Geometry check sheet. Reference: the model listing, model coordinates, mm. Face numbers are marked on the shaded views. Give positions to 0.01 mm unless a question says otherwise; leave off trailing zeros. Loops run counter-clockwise (first coordinate to the right, second up) from the corner with the lowest first, then second, coordinate; pieces in that order, holes last. Notation, with made-up numbers: (25, 20) -> (37, 20) arc R24 cw to (37, 50) -> close; hole circle Ø4 at (52, -32). An arc over 180 degrees is marked (long way). Write each question's results on one line, items separated by ' | '. Start each with the question number.
1) Scan lines: line 1 (X direction, y = -1.25, z = 12.5); line 2 (X direction, y = -4.5, z = -18.5); line 3 (Z direction, x = 14.5, y = -1.5). Record each from-to range of solid material in increasing order. Write a range as from..to.
2) Depth check by flat-ended pin: pin 1 (1 mm diameter, centred on y = -13, z = 52, fed in from -X); pin 2 (1.5 mm diameter, centred on x = -13.5, y = -8, fed in from +Z); pin 3 (6 mm diameter, centred on y = -4.5, z = 55, fed in from +X). Enter the tip coordinate at first touch or a pass-through.
3) Sectioned sample at C-C on x = 24. Record the cut outline in (y, z).
4) Sectioned sample at D-D on z = -1.5. Record the cut outline in (x, y).
5) Sectioned sample at A-A on z = 81.5. Record the cut outline in (x, y).
6) Draft check along X on the marked faces 1, 2 and 3. Enter one of: pulls with the +X half, pulls with the -X half, needs draft (parallel to the pull), parting line crosses it, or undercut.
7) Sectioned sample at B-B on y = -10.25. Record the cut outline in (x, z).
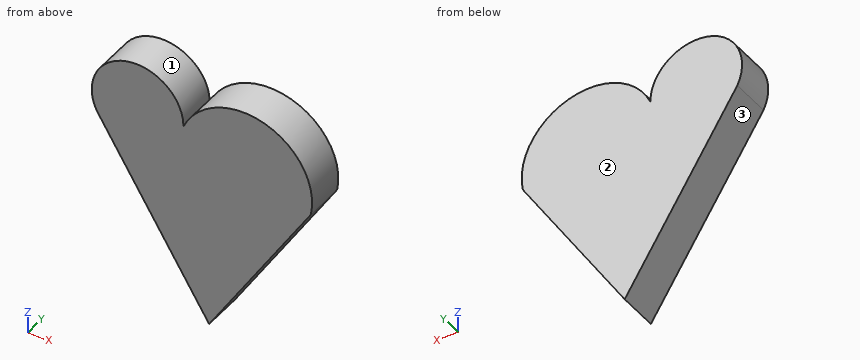
```python
from build123d import *

# Parameters (mm, degrees)
F1_DEPTH = 25.4


with BuildPart() as f1:
    # F0 (on Front) → F1 (new body)
    with BuildSketch(Plane.XZ):
        with BuildLine():
            ThreePointArc((51.010095, 54.163594), (21.668951, 102.782431), (-29.800825, 78.791678))
            Line((-29.800825, 78.791678), (-29.800825, 79.406742))
            ThreePointArc((-29.800825, 79.406742), (-65.60986, 107.361105), (-84.912881, 66.237792))
            Line((-84.912881, 66.237792), (-13.511168, -47.215126))
            Line((-13.511168, -47.215126), (51.010095, 54.163594))
        make_face()
        with BuildLine():
            Line((-29.800825, 79.406742), (-29.800825, 78.791678))
            ThreePointArc((-29.800825, 78.791678), (-29.799197, 79.09921), (-29.800825, 79.406742))
        make_face()
    extrude(amount=F1_DEPTH)


solid = f1.part
```
Result:
1) line 1: -51.09..24.49 | line 2: -31.58..4.76 | line 3: -3.2..104.31
2) pin 1: x = -76.27 | pin 2: z = 98.47 | pin 3: x = 51.56
3) outline: (-25.4, 11.72) -> (0, 11.72) -> (0, 102) -> (-25.4, 102) -> close
4) outline: (-42.28, -25.4) -> (15.58, -25.4) -> (15.58, 0) -> (-42.28, 0) -> close
5) outline: (-87.81, -25.4) -> (-29.9, -25.4) -> (-29.9, 0) -> (-87.81, 0) -> close; (-28.53, -25.4) -> (47.1, -25.4) -> (47.1, 0) -> (-28.53, 0) -> close
6) face 1: undercut | face 2: needs draft | face 3: pulls with the -X half
7) outline: (-84.91, 66.24) -> (-13.51, -47.22) -> (51.01, 54.16) arc R42.48 ccw to (-29.8, 78.79) arc R29.05 ccw to (-29.8, 79.41) arc R29.06 ccw (long way) to start
